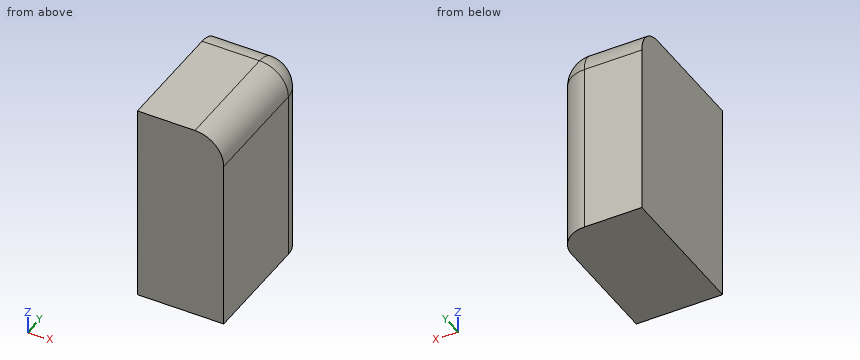
```python
from build123d import *

# Parameters (mm, degrees)
F0_W     = 30
F0_H     = 50
F1_DEPTH = 70
F3_R     = 10


# Not quite as in the source:
# - a feature of the source that left no trace in its solid (it failed there, or was rolled back) is left out


with BuildPart() as f1:
    # F0 (on Top) → F1 (new body)
    with BuildSketch(Plane.XY):
        with Locations((-0.0802149171, 25)):
            Rectangle(F0_W, F0_H)
    extrude(amount=F1_DEPTH)


with BuildPart() as f1_1:
    # F2: moved
    add(f1.part.moved(Location((30, 50, 70))))

    # F3
    f3_edges = [f1_1.edges().sort_by_distance(p)[0] for p in [
        (44.919785, 75, 140),
        (29.919785, 100, 140),
        (44.919785, 100, 105),
    ]]
    fillet(f3_edges, radius=F3_R)


solid = f1_1.part
```
Geometry check sheet. Reference: the model listing, model coordinates, mm. Round coordinates to 2 decimals unless told otherwise and drop trailing zeros. Order: outer loops, then holes, each group sorted by start corner. A loop starts at its lowest first (then second) coordinate and runs counter-clockwise, first axis right, second up. Notation, with made-up numbers: (64.25, 64.25) -> (115.25, 64.25) arc R21 cw to (115.25, 90.25) -> close; hole circle Ø3 at (67.25, 62.25). An arc over 180 degrees is marked (long way). Return JSON: item names as keys, results as strings. Group by question number.
Q1. Material ranges on probe 1 along X at (y, z) = (97, 122.5); probe 2 along Z at (x, y) = (43.25, 83); probe 3 along X at (y, z) = (72, 136), recorded low to high. Write a range as from..to.
Q2. Section check A-A, the plane x = 37.5. Record the boundary of the cut face in (y, z).
Q3. Section check B-B, the plane z = 132.5. Record the boundary of the cut face in (x, y).
Q4. Gauge pin test, flat end, axial feed: pin 1 (1.5 mm diameter, centred on x = 39, y = 57, fed in from +Z). Record the tip position at first contact, or that the pin passes through.
Numbers:
{
 "1": {"probe 1": "14.92..42.06", "probe 2": "70..135.53", "probe 3": "14.92..42.92"},
 "2": {"outline": "(50, 70) -> (99.66, 70) -> (99.66, 130) arc R9.66 ccw to (90, 139.66) -> (50, 139.66) -> close"},
 "3": {"outline": "(14.92, 50) -> (44.6, 50) -> (44.6, 90) arc R9.68 ccw to (34.92, 99.68) -> (14.92, 99.68) -> close"},
 "4": {"pin 1": "z = 139.43"}
}
